Autodesk Inventor part; units mm, degrees
ref_plane "Work Plane1" through (-2, -2, 15) normal (0, 0, 1) x (1, 0, 0)
ref_plane "YZ Plane" through (0, 0, 0) normal (1, 0, 0) x (0, 1, 0)
ref_plane "XZ Plane" through (0, 0, 0) normal (0, 1, 0) x (-1, 0, 0)
sketch "Sketch1" plane through (0, 0, 0) normal (0, 0, 1) x (1, 0, 0)
  line L0 (-2.4408, -0.5408) -> (-1.2026, 2.1918)
  arc A0 (-2.4408, -0.5408) -> (-1.2026, 2.1918) centre (0, 0) ccw
  circle A1 centre (0, 0) radius 3.5
  line L1 (-3.6608, -0.2297) -> (-3.4925, -0.2297)
  line L2 (-3.4925, 0.2297) -> (-3.6608, 0.2297)
  line L3 (-3.6608, 0.2297) -> (-3.6608, -0.2297)
  line L4 (-3.6608, -0.2297) -> (-3.5, 0) construction
  line L5 (-3.5, 0) -> (-3.6608, 0.2297) construction
  point P0 (0, 0)
  dimension "d0" = 7
ref_plane "Work Plane1" through (-2, -2, 15) normal (0, 0, 1) x (1, 0, 0)
extrude "Extrusion1" add sketch "Sketch1" along normal up to surface (15 mm away) contours A1
sketch "Sketch2" plane through (0, 0, 15) normal (0, 0, 1) x (1, 0, 0)
  arc A0 (-2.4408, -0.5408) -> (-1.2026, 2.1918) centre (0, 0) ccw
  line L0 (-1.2026, 2.1918) -> (-2.4408, -0.5408)
  circle A1 centre (0, 0) radius 3.5
  arc A2 (-2.702, -0.5115) -> (-1.3968, 2.3688) centre (0, 0) ccw
  line L1 (-2.702, -0.5115) -> (-1.3968, 2.3688)
  point P0 (0, 0)
  dimension "d9" = 0.25
extrude "Extrusion2" cut sketch "Sketch2" against normal up to surface (15 mm away) contours L1 A2
sketch "Sketch6" plane through (0, 0, 15) normal (0, 0, 1) x (1, 0, 0)
  circle A0 centre (0, 0) radius 10.15
  line L0 (0, 10.15) -> (8.7902, 5.075)
  line L1 (8.7902, 5.075) -> (8.7902, -5.075)
  line L2 (8.7902, -5.075) -> (0, -10.15)
  line L3 (0, -10.15) -> (-8.7902, -5.075)
  line L4 (-8.7902, -5.075) -> (-8.7902, 5.075)
  line L5 (-8.7902, 5.075) -> (0, 10.15)
  arc A1 (-2.702, -0.5115) -> (-1.3968, 2.3688) centre (0, 0) ccw
  line L6 (-1.3968, 2.3688) -> (-2.702, -0.5115)
  circle A2 centre (0, 0) radius 3.5
  point P0 (0, -10.15)
  point P1 (0, -10.15)
  dimension "d20" = 20.3
extrude "Extrusion5" add sketch "Sketch6" along normal blind 8 contours A0 L1 | L0 A0 | A0 L2 | L5 A0 | A0 L3 | L4 A0
extrude "Extrusion6" add sketch "Sketch6" against normal up to surface (15 mm away) contours A0 L1 | L0 A0 | L1 L2 L3 L4 L5 L0 | A0 L2 | L5 A0 | A0 L3 | L4 A0
sketch "Sketch7" plane through (0, 0, 0) normal (0, 0, -1) x (-1, 0, 0)
  circle A0 centre (0, 0) radius 10.15
  arc A1 (1.3968, 2.3688) -> (2.702, -0.5115) centre (0, 0) ccw
  line L0 (1.3968, 2.3688) -> (2.702, -0.5115)
  circle A2 centre (0, 0) radius 11.15
  dimension "d25" = 1
extrude "Extrusion7" add sketch "Sketch7" against normal up to surface (23 mm away) contours A2
sketch "Sketch8" plane through (0, 0, 23) normal (0, 0, 1) x (1, 0, 0)
  circle A0 centre (0, 0) radius 11.15
  line L0 (-8.7902, -5.075) -> (-8.7902, 5.075)
  line L1 (-8.7902, 5.075) -> (0, 10.15)
  line L2 (0, 10.15) -> (8.7902, 5.075)
  line L3 (8.7902, 5.075) -> (8.7902, -5.075)
  line L4 (8.7902, -5.075) -> (0, -10.15)
  line L5 (0, -10.15) -> (-8.7902, -5.075)
  point P0 (0, 0)
extrude "Extrusion8" add sketch "Sketch8" along normal blind 8
properties part number "RodMotorMount"
Read the model definition and answer for the solid it produces. Units are mm, in the model's axes. A direction names the side the tool comes from. Coordinates: 2 decimals unless noted, no trailing zeros. Loops run counter-clockwise (first coordinate to the right, second up) from the corner with the lowest first, then second, coordinate; pieces in that order, holes last.
Q1. Which of the six approach directions +Z, -Z, +X, -X, +Y, -Y give full straight-line access (tool end or side, diameter ignored) to faces 4 (the face through (-4.457, 7.577, 22.888)), 5 (the face through (-2.3, -2.3, 0)), 6 (the face through (-2.06, 0.91, 7.6))?
Q2. The part is cut by section D-D on y = -3.25. Write down the section's boundary in (x, z).
Q3. Consider probe 1 along Z at (x, y) = (4.5, 6.5); probe 2 along X at (y, z) = (3.25, 16.5); probe 3 along Y at (x, z) = (1.25, 8). Determine where each line is inside the solid, lowest interval first.
Q4. The mould has two halves that part along X. Classify faces 1 (the face through (-0.735, 11.126, 15.283)), 2 (the face through (4.1, -8.2, 31)), 3 (the face through (4.457, -7.577, 22.888)): +X half, -X half, draft (parallel to the pull), parting line (faces both ways), or undercut.
Q5. The part is cut by section A-A on z = 28. Write down the section's boundary in (x, y) (3 decimals), and give its area (3 significant figures).
Q6. Each of these flat-tipped pins is pushed along its axis until it touches: pin 1 Ø8 at (y, z) = (3.5, 27) entering from +X; pin 2 Ø5 at (x, z) = (-3, 12) entering from +Y; pin 3 Ø3 at (y, z) = (-3.5, 27) entering from -X; pin 4 Ø4 at (y, z) = (-7, 10.5) entering from +X. Where does it stop, or does it pass through?
Q7. The part is cut by section C-C on x = 5.25. Write down the section's boundary in (y, z).
Q8. The part is cut by section B-B on y = 0. Write down the section's boundary in (x, z).
Results below:
1. face 4: +Z
1. face 5: -Z, +X, -X, +Y, -Y
1. face 6: +Z, -Z
2. outline: (-10.67, 0) - (10.67, 0) - (10.67, 31) - (8.79, 31) - (8.79, 15) - (-8.79, 15) - (-8.79, 31) - (-10.67, 31) - close
3. probe 1: z = 0 to 15
3. probe 2: x = -10.67 to -8.79, 8.79 to 10.67
3. probe 3: y = -11.08 to -2.45, 2.45 to 11.08
4. face 1: parting line
4. face 2: draft
4. face 3: undercut
5. outline: circle Ø22.3 at (0, 0); hole (-8.79, -5.075) - (0, -10.15) - (8.79, -5.075) - (8.79, 5.075) - (0, 10.15) - (-8.79, 5.075) - close
5. area: 123 mm2
6. pin 1: stops at x = 11.15
6. pin 2: stops at y = 11.14
6. pin 3: stops at x = -10.97
6. pin 4: stops at x = 9.97
7. outline: (-9.84, 0) - (9.84, 0) - (9.84, 31) - (7.12, 31) - (7.12, 15) - (-7.12, 15) - (-7.12, 31) - (-9.84, 31) - close
8. outline: (-11.15, 0) - (-2.47, 0) - (-2.47, 15) - (-8.79, 15) - (-8.79, 31) - (-11.15, 31) - close; (2.75, 0) - (11.15, 0) - (11.15, 31) - (8.79, 31) - (8.79, 15) - (2.75, 15) - close
